Part model, mm, in its own coordinate system. Face numbers are marked on the shaded views. A direction names the side the tool comes from. Round coordinates to 2 decimals unless told otherwise and drop trailing zeros. Write each loop counter-clockwise with the first axis right and the second up, starting at its lowest first coordinate (ties: lowest second). Pieces come first, ordered by that corner, then holes. Notation, with made-up numbers: M 60.5,54 L 111.5,54 A16 ccw 111.5,79 Z; hole C 43,48.25 d3. An arc over 180 degrees is marked long. Answer as a JSON object with one key per item and string values. Group by question number.
1. Two-plate mould, pull along Y, no slides. Class the marked faces 4, 5 and 6: +Y half, -Y half, draft (parallel to the pull), parting line (faces both ways), or undercut.
2. Band-saw the part on A-A, the plane z = 113. Write the cut outline in (x, y), plus the area to 3 significant figures.
3. Band-saw the part on B-B, the plane x = 78. Write the cut outline in (y, z).
4. Drill centre lines: line 1 (X direction, y = -161, z = 33); line 2 (X direction, y = -68.5, z = 14); line 3 (Y direction, x = 95, z = 76.5). Where is each one in solid material? Low to high. Write a range as from..to.
5. Which spindle directions (+Z, -Z, +X, -X, +Y, -Y) get a long thin tool onto all of the face, cutting with end or side? Do the marked faces 1, 2 and 3. Say none if no direction does.
6. Drop flat-ended pins along their axis: pin 1 (17.5 mm diameter, centred on y = -59, z = 56, fed in from -X); pin 2 (3.5 mm diameter, centred on x = 69.5, y = -132, fed in from +Z); pin 3 (5 mm diameter, centred on y = -93, z = 35.5, fed in from -X). Give the stop position or say it passes through.
7. Band-saw the part on C-C, the plane y = -101.5. Write the cut outline in (x, z), plus the area to 3 significant figures.
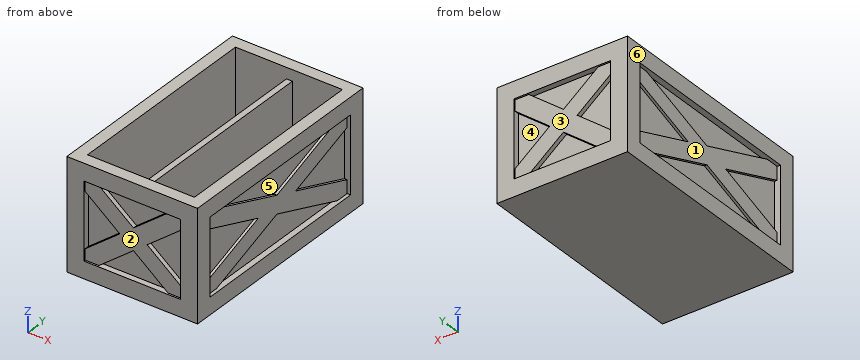
from build123d import *

# Parameters (mm, degrees)
F0_W      = 140
F0_H      = 130
F1_DEPTH  = 250
F2_W      = 126
F2_H      = 236
F3_DEPTH  = 123
F4_W      = 250
F4_H      = 130
F4_W_2    = 224
F4_H_2    = 90
F4_W_3    = 7
F5_DEPTH  = 7
F7_W      = 140
F7_H      = 130
F7_W_2    = 114
F7_H_2    = 90
F8_DEPTH  = 7
F9_W      = 140
F9_H      = 130
F9_W_2    = 114
F9_H_2    = 90
F10_DEPTH = 7
F12_DEPTH = 3
F14_DEPTH = 3
F15_W     = 7
F15_H     = 110
F16_DEPTH = 236
F18_DEPTH = 5


# Not quite as in the source:
# - a pattern or mirror of a feature is missing from the dataset's text; its kind, count and spacing are read off the source's solid


with BuildPart() as f1:
    # F0 (on Front) → F1 (new body)
    with BuildSketch(Plane.XZ):
        with Locations((70, 65)):
            Rectangle(F0_W, F0_H)
    extrude(amount=F1_DEPTH)

    # F2 (on face) → F3 (cut)
    with BuildSketch(Plane.XY.offset(130)):
        with Locations((70, -125)):
            Rectangle(F2_W, F2_H)
    extrude(amount=-F3_DEPTH, mode=Mode.SUBTRACT)

    # F4 (on face) → F5 (join)
    with BuildSketch(Plane.YZ.offset(140)):
        with Locations((-125, 65)):
            Rectangle(F4_W, F4_H)
        with Locations((-125, 65)):
            Rectangle(F4_W_2, F4_H_2, mode=Mode.SUBTRACT)
        with Locations((-253.5, 65)):
            Rectangle(F4_W_3, F4_H)
        with Locations((3.5, 65)):
            Rectangle(F4_W_3, F4_H)
    f5 = extrude(amount=F5_DEPTH)

    # F5_copies: F5 across plane
    add(f5.mirror(Plane(origin=(70, 0, 0), x_dir=(0, 0, -1), z_dir=(-1, 0, 0))))

    # F7 (on face) → F8 (join)
    with BuildSketch(Plane.XZ.offset(250)):
        with Locations((70, 65)):
            Rectangle(F7_W, F7_H)
        with Locations((70, 65)):
            Rectangle(F7_W_2, F7_H_2, mode=Mode.SUBTRACT)
    extrude(amount=F8_DEPTH)

    # F9 (on face) → F10 (join)
    with BuildSketch(Plane(origin=(0, 0, 0), x_dir=(-1, 0, 0), z_dir=(0, 1, 0))):
        with Locations((-70, 65)):
            Rectangle(F9_W, F9_H)
        with Locations((-70, 65)):
            Rectangle(F9_W_2, F9_H_2, mode=Mode.SUBTRACT)
    extrude(amount=F10_DEPTH)

    # F11 (on face) → F12 (join)
    with BuildSketch(Plane.YZ.offset(140)):
        Polygon((-13, 35.6504185324), (-221.3495814676, 110), (-237, 110), (-237, 94.3495814676), (-28.6504185324, 20), (-13, 20), align=None)
    f12 = extrude(amount=F12_DEPTH)

    # F12_copies: F12 across plane
    add(f12.mirror(Plane(origin=(70, 0, 0), x_dir=(0, 0, -1), z_dir=(-1, 0, 0))))

    # F13 (on face) → F14 (join)
    with BuildSketch(Plane.YZ.offset(140)):
        Polygon((-13, 110), (-28.6504185324, 110), (-237, 35.6504185324), (-237, 20), (-221.3495814676, 20), (-13, 94.3495814676), align=None)
    f14 = extrude(amount=F14_DEPTH)

    # F14_copies: F14 across plane
    add(f14.mirror(Plane(origin=(70, 0, 0), x_dir=(0, 0, -1), z_dir=(-1, 0, 0))))

    # F15 (on face) → F16 (join, through all)
    with BuildSketch(Plane.XZ.offset(7)):
        with Locations((70.5, 62)):
            Rectangle(F15_W, F15_H)
    extrude(amount=F16_DEPTH)

    # F17 (on face) → F18 (join)
    with BuildSketch(Plane.XZ.offset(250)):
        Polygon((70, 77.7407562494), (29.1382912492, 110), (13, 110), (13, 97.2592437506), (53.8617087508, 65), (13, 32.7407562494), (13, 20), (29.1382912492, 20), (70, 52.2592437506), (110.8617087508, 20), (127, 20), (127, 32.7407562494), (86.1382912492, 65), (127, 97.2592437506), (127, 110), (110.8617087508, 110), align=None)
    f18 = extrude(amount=F18_DEPTH)

    # F18_copies: F18 across plane
    add(f18.mirror(Plane.ZX.offset(-125)))


solid = f1.part
Worked answers:
{
 "1": {"face 4": "+Y half", "face 5": "undercut", "face 6": "draft"},
 "2": {"outline": "M -7,-257 L 147,-257 L 147,7 L -7,7 Z; hole M 7,-243 L 67,-243 L 67,-7 L 7,-7 Z; hole M 74,-243 L 133,-243 L 133,-7 L 74,-7 Z", "area": "12,600 mm^2"},
 "3": {"outline": "M -257,0 L 7,0 L 7,20 L 0,20 L 0,45.94 L 5,45.94 L 5,84.06 L 0,84.06 L 0,110 L 7,110 L 7,130 L -7,130 L -7,7 L -243,7 L -243,130 L -257,130 L -257,110 L -250,110 L -250,84.06 L -255,84.06 L -255,45.94 L -250,45.94 L -250,20 L -257,20 Z"},
 "4": {"line 1": "x = 0..7, 67..74, 133..140", "line 2": "x = -7..7, 67..74, 133..147", "line 3": "y = -255..-243, -7..5"},
 "5": {"face 1": "-X", "face 2": "-Y", "face 3": "+Y"},
 "6": {"pin 1": "stops at x = -3", "pin 2": "stops at z = 117", "pin 3": "stops at x = 0"},
 "7": {"outline": "M -7,0 L 147,0 L 147,20 L 140,20 L 140,46 L 143,46 L 143,84 L 140,84 L 140,110 L 147,110 L 147,130 L 133,130 L 133,7 L 74,7 L 74,117 L 67,117 L 67,7 L 7,7 L 7,130 L -7,130 L -7,110 L 0,110 L 0,84 L -3,84 L -3,46 L 0,46 L 0,20 L -7,20 Z", "area": "4,260 mm^2"}
}
